```python
from build123d import *

# Parameters (mm, degrees)
ESBO_O1_R                = 6
RESSALTO_EXTRUS_O1_DEPTH = 35
CHANFRO1_SIZE            = 2
ESBO_O2_R                = 3.4
CORTE_EXTRUS_O1_DEPTH    = 25


with BuildPart() as part:
    # Esboço1 → Ressalto-extrusão1 (new body)
    with BuildSketch(Plane(origin=(0, 0, 0), x_dir=(1, 0, 0), z_dir=(0, 1, 0))):
        with Locations(Location((0, 0, 0), (0, 0, 270))):
            Circle(ESBO_O1_R)
    extrude(amount=RESSALTO_EXTRUS_O1_DEPTH)

    # Chanfro1
    chanfro1_edges = [part.edges().sort_by_distance(p)[0] for p in [
        (0, 35, -6),
    ]]
    chamfer(chanfro1_edges, length=CHANFRO1_SIZE)

    # Esboço2 → Corte-extrusão1 (cut)
    with BuildSketch(Plane.XZ):
        with Locations(Location((0, 0, 0), (0, 0, 270))):
            Circle(ESBO_O2_R)
    extrude(amount=-CORTE_EXTRUS_O1_DEPTH, mode=Mode.SUBTRACT)


solid = part.part
```
Design review of the part built by this model. Coordinates are the model's own, in mm. A direction names the side the tool comes from. Coordinates: 2 decimals unless noted, no trailing zeros. Write each loop counter-clockwise with the first axis right and the second up, starting at its lowest first coordinate (ties: lowest second). Pieces come first, ordered by that corner, then holes.
1) Add section D-D (y = 20). Write out the cut boundary in (x, z), plus the area to 3 significant figures.
2) Insertion check: pin 1 (6 mm diameter, centred on y = 20, z = 3.5, fed in from -X); pin 2 (1.5 mm diameter, centred on y = 4.5, z = -3, fed in from +X); pin 3 (3 mm diameter, centred on y = 30.5, z = 3.5, fed in from -X). Each pin has a flat end and moves straight along its axis. Give the tip position at first contact, or say it passes through.
3) Mouldability with a two-part tool opening along Z and no side actions: class faces 1 (the cylindrical face through (1.802, 16.269, 5.723)), 2 (the flat face through (0, 25, 0)), 3 (the flat face through (0, 35, 0)) as +Z half, -Z half, draft (parallel to the pull), parting line (faces both ways), or undercut.
4) Add section A-A (x = 0). Write out the cut boundary in (y, z).
5) Machinability: for faces 4 (the cylindrical face through (-3.32, 12.32, 0.74)), 5 (the flat face through (-3, 0, 3)), which of the approach directions +Z, -Z, +X, -X, +Y, -Y give a long, thin tool a straight path to every point of the face, cutting with its end or side? Answer none if there is none.
6) Add section B-B (z = 0). Write out the cut boundary in (x, y), plus the area to 3 significant figures.
7) Add section C-C (y = 27.5). Write out the cut boundary in (x, z).
8) To check wall thickness, follow L1, parallel to X at y = 10.5, z = 0; L2, parallel to Y at x = -0.75, z = 0.25; L3, parallel to X at y = 14.5, z = -1. State the ranges of each line that lie inside material, in increasing order.
Check result:
1. outline: circle Ø12 at (0, 0); hole circle Ø6.8 at (0, 0)
1. area: 76.8 mm2
2. pin 1: stops at x = -5.98
2. pin 2: stops at x = 5.56
2. pin 3: stops at x = -5.66
3. face 1: parting line
3. face 2: undercut
3. face 3: draft
4. outline: (0, -6) - (33, -6) - (35, -4) - (35, 4) - (33, 6) - (0, 6) - (0, 3.4) - (25, 3.4) - (25, -3.4) - (0, -3.4) - close
5. face 4: -Y
5. face 5: +Z, -Z, +X, -X, -Y
6. outline: (-6, 0) - (-3.4, 0) - (-3.4, 25) - (3.4, 25) - (3.4, 0) - (6, 0) - (6, 33) - (4, 35) - (-4, 35) - (-6, 33) - close
6. area: 246 mm2
7. outline: circle Ø12 at (0, 0)
8. L1: x = -6 to -3.4, 3.4 to 6
8. L2: y = 25 to 35
8. L3: x = -5.92 to -3.25, 3.25 to 5.92
